Source: three-view drawing plus pictorial views. Frame: mm from the lowest corner of the part. A direction names the side the tool comes from. Give positions to 0.01 mm unless a question says otherwise; leave off trailing zeros. Order: outer loops, then holes, each group sorted by start corner. A loop starts at its lowest first (then second) coordinate and runs counter-clockwise, first axis right, second up. Notation, with made-up numbers: (-32, -0.5) -> (-14, -0.5) arc R32 ccw to (-14, 29.5) -> close; hole circle Ø2 at (-13, -37.5). An arc over 180 degrees is marked (long way). One line per question, with ' | ' between items.
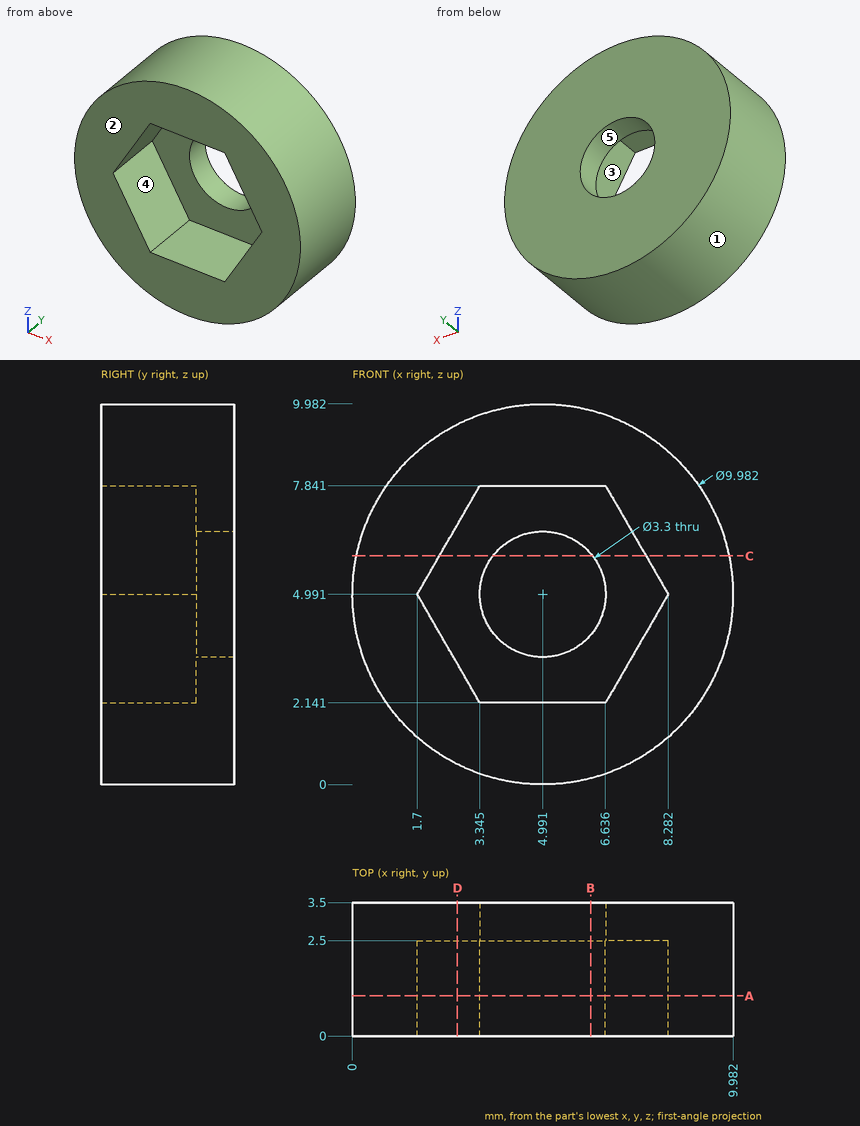
1) Set-up query: the marked faces 4 and 5. Return all of +Z, -Z, +X, -X, +Y, -Y with unobstructed straight access to the full face (end or side cutting, diameter ignored); none if empty.
Check result:
face 4: -Y | face 5: +Y, -Y
2) Contact query for flat-ended pins moving along their axis: pin 1 Ø0.8 at (x, y) = (4, 1) entering from -Z (1 decimal); pin 2 Ø2 at (x, y) = (2.5, 1.5) entering from -Z; pin 3 Ø1 at (x, y) = (6, 1.5) entering from +Z. Output: stop coordinate, or through.
Check result:
pin 1: stops at z = 0 | pin 2: stops at z = 0.23 | pin 3: stops at z = 9.96
3) Section D-D on x = 2.75. Return loops of the section in (y, z).
Check result:
outline: (0, 0.53) -> (3.5, 0.53) -> (3.5, 9.45) -> (0, 9.45) -> (0, 6.81) -> (2.5, 6.81) -> (2.5, 3.17) -> (0, 3.17) -> close
4) Section A-A on y = 1.05. Return loops of the section in (x, z) (1 decimal).
Check result:
outline: circle Ø10 at (5, 5); hole (1.7, 5) -> (3.3, 2.1) -> (6.6, 2.1) -> (8.3, 5) -> (6.6, 7.8) -> (3.3, 7.8) -> close
5) Pull-direction query (Z, two-part tool) for the marked faces 1, 2 and 3; classes: +Z half, -Z half, draft (parallel to the pull), parting line (faces both ways), or undercut.
Check result:
face 1: parting line | face 2: draft | face 3: undercut
6) Material intervals for probe 1 along X at (y, z) = (2.8, 3.75) (1 decimal); probe 2 along X at (y, z) = (2.05, 4.25) (1 decimal); probe 3 along Z at (x, y) = (4.5, 0.4) (1 decimal), sorted ascending. Write a range as from..to.
Check result:
probe 1: x = 0.2..3.9, 6.1..9.8 | probe 2: x = 0.1..2.1, 7.9..9.9 | probe 3: z = 0..2.1, 7.8..10
7) Section B-B on x = 6.25. Return loops of the section in (y, z) (1 decimal).
Check result:
outline: (0, 0.2) -> (3.5, 0.2) -> (3.5, 3.9) -> (2.5, 3.9) -> (2.5, 2.1) -> (0, 2.1) -> close; (0, 7.8) -> (2.5, 7.8) -> (2.5, 6.1) -> (3.5, 6.1) -> (3.5, 9.8) -> (0, 9.8) -> close
8) Section C-C on z = 6. Return loops of the section in (x, y) (1 decimal).
Check result:
outline: (0.1, 0) -> (2.3, 0) -> (2.3, 2.5) -> (3.7, 2.5) -> (3.7, 3.5) -> (0.1, 3.5) -> close; (6.3, 2.5) -> (7.7, 2.5) -> (7.7, 0) -> (9.9, 0) -> (9.9, 3.5) -> (6.3, 3.5) -> close
